Read the model definition and answer for the solid it produces. Units are mm, in the model's axes. A direction names the side the tool comes from. Coordinates: 2 decimals unless noted, no trailing zeros. Loops run counter-clockwise (first coordinate to the right, second up) from the corner with the lowest first, then second, coordinate; pieces in that order, holes last.
from build123d import *

# Parameters (mm, degrees)
SKETCH1_R                        = 15.8369
EXTRUDE1_DEPTH                   = 25.4
SKETCH2_W                        = 66.04
SKETCH2_H                        = 34.925
EXTRUDE2_DEPTH                   = 12.7
SKETCH4_R                        = 6.35
CUT_EXTRUDE1_DEPTH               = 70.85
SKETCH6_R                        = 9.525
CUT_EXTRUDE5_DEPTH               = 8.89
SKETCH7_W                        = 18.923
SKETCH7_H                        = 18.923
SKETCH7_R                        = 6.35
EXTRUDE3_DEPTH                   = 6.35
SKETCH9_OUTSIDE_W                = 88.494
SKETCH9_OUTSIDE_H                = 57.38
SKETCH9_OUTSIDE_R                = 10.414
CUT_EXTRUDE7_DEPTH               = 6.35
FILLET1_R                        = 12.7
F_1_4_20_TAPPED_HOLE1_D          = 5.1054
F_13_32_0_40625_DIAMETER_HOLE1_D = 10.31875
CHAMFER2_SIZE                    = 1.524


with BuildPart() as part:
    # Sketch1 → Extrude1 (new body)
    with BuildSketch(Plane.XY):
        Circle(SKETCH1_R)
    extrude(amount=EXTRUDE1_DEPTH)

    # Sketch2 → Extrude2 (add)
    with BuildSketch(Plane.XY.offset(25.4)):
        Rectangle(SKETCH2_W, SKETCH2_H)
    extrude(amount=EXTRUDE2_DEPTH)

    # Sketch3 → Revolve1 (revolve)
    with BuildSketch(Plane(origin=(0, 0, 0), x_dir=(1, 0, 0), z_dir=(0, 1, 0))):
        Polygon((0, 0), (0, 31.75), (9.4615, 31.75), (9.4615, 25.4), (15.8369, 25.4), (15.8369, 0), align=None)
    revolve(axis=Axis((0, 0, 0), (0, 0, -1)))

    # Sketch4 → Cut-Extrude1 (cut, through all)
    with BuildSketch(Plane.XY.offset(38.1)):
        Circle(SKETCH4_R)
    extrude(amount=-CUT_EXTRUDE1_DEPTH, mode=Mode.SUBTRACT)

    # Sketch6 → Cut-Extrude5 (cut)
    with BuildSketch(Plane.XY.offset(38.1)):
        Circle(SKETCH6_R)
    extrude(amount=-CUT_EXTRUDE5_DEPTH, mode=Mode.SUBTRACT)

    # Sketch7 → Extrude3 (add)
    with BuildSketch(Plane(origin=(0, 0, -25.4), x_dir=(-1, 0, 0), z_dir=(0, 0, -1))):
        Rectangle(SKETCH7_W, SKETCH7_H)
        with Locations(Location((0, 0, 0), (0, 0, 180))):  # turned: the seam where the file's is
            Circle(SKETCH7_R, mode=Mode.SUBTRACT)
    extrude(amount=EXTRUDE3_DEPTH)

    # Sketch9 outside → Cut-Extrude7 (cut)
    with BuildSketch(Plane(origin=(0, 0, -31.75), x_dir=(-1, 0, 0), z_dir=(0, 0, -1))):
        Rectangle(SKETCH9_OUTSIDE_W, SKETCH9_OUTSIDE_H)
        Circle(SKETCH9_OUTSIDE_R, mode=Mode.SUBTRACT)
    extrude(amount=-CUT_EXTRUDE7_DEPTH, mode=Mode.SUBTRACT)

    # Fillet1
    fillet1_edges = [part.edges().sort_by_distance(p)[0] for p in [
        (-33.02, 17.4625, 31.75),
        (-33.02, -17.4625, 31.75),
        (33.02, -17.4625, 31.75),
        (33.02, 17.4625, 31.75),
    ]]
    fillet(fillet1_edges, radius=FILLET1_R)

    # 1/4-20 Tapped Hole1 (through all)
    with Locations(Plane.XY.offset(38.1)):
        with Locations((18.288, -10.9855), (-18.288, 10.9855)):
            Hole(F_1_4_20_TAPPED_HOLE1_D / 2)

    # 13/32 (0.40625) Diameter Hole1 (through all)
    with Locations(Plane.XY.offset(38.1)):
        with Locations((-23.8125, 0), (23.8125, 0)):
            Hole(F_13_32_0_40625_DIAMETER_HOLE1_D / 2)

    # Chamfer2
    chamfer2_edges = [part.edges().sort_by_distance(p)[0] for p in [
        (9.4615, 0, -31.75),
        (-9.4615, 0, -31.75),
    ]]
    chamfer(chamfer2_edges, length=CHAMFER2_SIZE)


solid = part.part
Q1. A cutting plane is placed at D-D (z = -9.5). Give the vertices of the cut face in (x, y), then the cut area to 3 significant figures.
Findings below:
outline: circle Ø31.67 at (0, 0); hole circle Ø12.7 at (0, 0)
area: 661 mm2
Q2. A cutting plane is placed at C-C (z = 26.5). Give the vertices of the cut face in (x, y).
Findings below:
outline: (-33.02, -4.76) arc R12.7 ccw to (-20.32, -17.46) - (20.32, -17.46) arc R12.7 ccw to (33.02, -4.76) - (33.02, 4.76) arc R12.7 ccw to (20.32, 17.46) - (-20.32, 17.46) arc R12.7 ccw to (-33.02, 4.76) - close; hole circle Ø10.32 at (-23.81, 0); hole circle Ø5.11 at (-18.29, 10.99); hole circle Ø12.7 at (0, 0); hole circle Ø5.11 at (18.29, -10.99); hole circle Ø10.32 at (23.81, 0)
Q3. Straight lines are drawn through the part: probe 1 along Y at (x, z) = (0, 35) (1 decimal); probe 2 along Y at (x, z) = (0, -13); probe 3 along Z at (x, y) = (28.5, -12). For each, find the intervals that lie inside material, in ascending order.
Findings below:
probe 1: y = -17.5 to -9.5, 9.5 to 17.5
probe 2: y = -15.84 to -6.35, 6.35 to 15.84
probe 3: z = 25.4 to 38.1
Q4. A cutting plane is placed at B-B (y = 0). Count the separate pieces of the cut face and the enclosed holes in it, then the cut area to 3 significant figures.
Findings below:
separate pieces: 4
enclosed holes: 0
area: 1,360 mm2
Q5. Which of the six approach directions +Z, -Z, +X, -X, +Y, -Y give full straight-line access (tool end or side, diameter ignored) to faces 1 (the face through (-7.4, 7.33, -28.62)), 2 (the face through (7.33, 7.4, -28.62)), 3 (the face through (-9.462, 0, -28))?
Findings below:
face 1: -Z, -X, +Y
face 2: -Z, +X, +Y
face 3: -Z, -X, +Y, -Y
Q6. Flat-ended cylindrical pins translate along their axes: pin 1 Ø10 at (x, z) = (18.5, 13) entering from +Y; pin 2 Ø17 at (x, y) = (0, 0) entering from +Z; pin 3 Ø12 at (x, z) = (-12, 9) entering from +Y; pin 4 Ø9.5 at (x, y) = (-23.81, 0) entering from +Z. Find the tip coordinate at first contact, or state that the pin passes through.
Findings below:
pin 1: stops at y = 8.28
pin 2: stops at z = 29.21
pin 3: stops at y = 14.66
pin 4: passes through
